```python
from build123d import *

# Parameters (mm, degrees)
F0_W          = 30.48
F0_H          = 15.24
F1_DEPTH      = 88.9
F2_W          = 30.48
F2_H          = 15.24
F3_DEPTH      = 38.1
F4_W          = 30.48
F4_H          = 15.24
F5_DEPTH      = 38.1
F6_R          = 3.81
F7_DEPTH      = 127
F7_DEPTH_BACK = 38.1
F9_DEPTH      = 88.9
F10_W         = 66.04
F10_H         = 73.66
F11_DEPTH     = 25.4
F12_W         = 63.5
F12_H         = 25.4
F13_DEPTH     = 12.7
F15_W         = 76.2
F15_H         = 25.4
F16_DEPTH     = 50.8
F18_DEPTH     = 7.62
F19_W         = 26.801726786
F19_H         = 6.35
F14_W         = 25.4
F14_H         = 6.35
F20_DEPTH     = 12.7
F21_DEPTH     = 12.7
F22_W         = 50.8
F22_H         = 25.4
F23_DEPTH     = 38.1
F24_DEPTH     = 12.7


# Not quite as in the source:
# - a feature names something its author has since deleted; it is built from what else it names


with BuildPart() as f1:
    # F0 (on Front) → F1 (new body)
    with BuildSketch(Plane.XZ):
        Polygon((0, 50.8), (0, 0), (29.5417681336, 0), (29.5417681336, 15.24), (60.0217681336, 15.24), (60.0217681336, 0), (121.1203709245, 0), (121.1203709245, 15.24), (151.6003709245, 15.24), (151.6003709245, 0), (203.2, 0), (203.2, 41.0980633142), (127, 41.0980633142), (127, 79.1980633142), (63.5, 79.1980633142), (38.1, 50.8), align=None)
        with Locations((44.7817681336, 7.62)):
            Rectangle(F0_W, F0_H)
        with Locations((136.3603709245, 7.62)):
            Rectangle(F0_W, F0_H)
    extrude(amount=F1_DEPTH)

    # F2 (on face) → F3 (cut)
    with BuildSketch(Plane.XZ.offset(88.9)):
        with Locations((45.8910012597, 7.62)):
            Rectangle(F2_W, F2_H)
        with Locations((127.1710012597, 7.62)):
            Rectangle(F2_W, F2_H)
    extrude(amount=-F3_DEPTH, mode=Mode.SUBTRACT)

    # F4 (on face) → F5 (cut)
    with BuildSketch(Plane(origin=(0, 0, 0), x_dir=(-1, 0, 0), z_dir=(0, 1, 0))):
        with Locations((-126.0602, 7.62)):
            Rectangle(F4_W, F4_H)
        with Locations((-44.7802, 7.62)):
            Rectangle(F4_W, F4_H)
    extrude(amount=-F5_DEPTH, mode=Mode.SUBTRACT)

    # F6 (on Front) → F7 (join, two sides)
    with BuildSketch(Plane.XZ) as f7_sk:
        with Locations((53.3541933731, 7.3445781872)):
            Circle(F6_R)
        with Locations((117.9336786941, 6.9635785541)):
            Circle(F6_R)
    extrude(amount=F7_DEPTH)
    extrude(f7_sk.sketch, amount=-F7_DEPTH_BACK)

    # F8 (on Front) → F9 (cut)
    with BuildSketch(Plane.XZ):
        Polygon((69.4312418273, 74.989986462), (44.0312418273, 46.5919231478), (82.1312418273, 46.5919231478), (82.1312418273, 74.989986462), align=None)
    extrude(amount=F9_DEPTH, mode=Mode.SUBTRACT)

    # F10 (on face) → F11 (cut)
    with BuildSketch(Plane.XY.offset(41.0980633142)):
        with Locations((160.02, -44.45)):
            Rectangle(F10_W, F10_H)
    extrude(amount=-F11_DEPTH, mode=Mode.SUBTRACT)

    # F12 (on face) → F13 (cut)
    with BuildSketch(Plane(origin=(-4.0760562793, 0, 3.6457355683), x_dir=(0, -1, 0), z_dir=(-0.7453559925, 0, 0.6666666667))):
        with Locations((43.8565216027, 81.8850251743)):
            Rectangle(F12_W, F12_H)
    extrude(amount=-F13_DEPTH, mode=Mode.SUBTRACT)

    # F15 (on face) → F16 (cut)
    with BuildSketch(Plane.YZ.offset(127)):
        with Locations((-44.45, 60.8695521951)):
            Rectangle(F15_W, F15_H)
    extrude(amount=-F16_DEPTH, mode=Mode.SUBTRACT)

    # F17 (on face) → F18 (join)
    with BuildSketch(Plane(origin=(0, 0, 0), x_dir=(0, -1, 0), z_dir=(-1, 0, 0))):
        Polygon((56.9462627172, 26.2763872743), (56.9462627172, 31.5944552422), (37.3661071062, 31.5944552422), (37.3661071062, 26.0346587747), (24.7961338609, 26.0346587747), (27.4551659822, 18.7827479094), (37.6078411937, 18.7827479094), (37.6078411937, 13.9481425285), (56.7045323551, 13.9481425285), (56.7045323551, 18.7827479094), (68.0658593774, 18.7827479094), (63.7147128582, 26.2763872743), align=None)
    extrude(amount=-F18_DEPTH)

    # F19 (on face) + F14 (on face) → F20 (join)
    with BuildSketch(Plane(origin=(0, 0, 0), x_dir=(0, -1, 0), z_dir=(-1, 0, 0))):
        with Locations((70.2801537674, 38.6348730328)):
            Rectangle(F19_W, F19_H)
    with BuildSketch(Plane(origin=(0, 0, 0), x_dir=(0, -1, 0), z_dir=(-1, 0, 0))):
        with Locations((18.7792903744, 38.6348730328)):
            Rectangle(F14_W, F14_H)
    extrude(amount=F20_DEPTH)

    # F21 (cut): faces of the model
    f21_faces = [f1.faces().sort_by_distance(p)[0] for p in [
        (-12.7, -18.7792903744, 38.6348730328),
        (-12.7, -70.2801537674, 38.6348730328),
    ]]
    extrude(f21_faces, amount=-F21_DEPTH, mode=Mode.SUBTRACT)

    # F22 (on face) → F23 (join)
    with BuildSketch(Plane.YZ.offset(127)):
        with Locations((-45.72, 28.3980633142)):
            Rectangle(F22_W, F22_H)
    extrude(amount=F23_DEPTH)

    # F24 (cut): a face of the model
    f24_faces = [f1.faces().sort_by_distance(p)[0] for p in [
        (165.1, -45.72, 28.3980633142),
    ]]
    extrude(f24_faces, amount=-F24_DEPTH, mode=Mode.SUBTRACT)


solid = f1.part
```
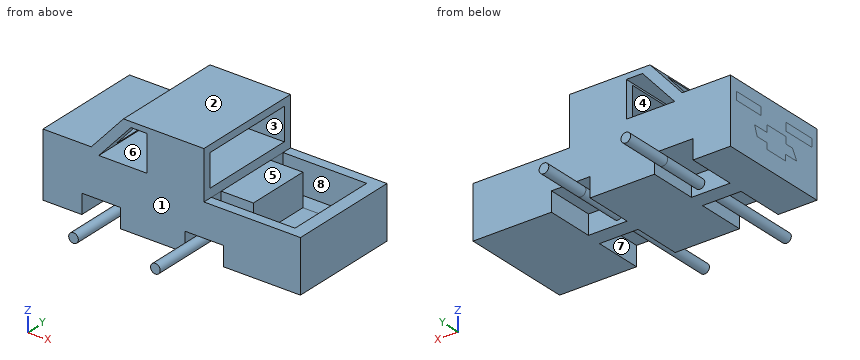
Can you work these out from the model? Positions are in its coordinate system, mm. Face numbers are marked on the shaded views. A direction names the side the tool comes from. Coordinates: 2 decimals unless noted, no trailing zeros. Order: outer loops, then holes, each group sorted by start corner. A loop starts at its lowest first (then second) coordinate and runs counter-clockwise, first axis right, second up. Notation, with made-up numbers: (48.5, 3.25) - (52.5, 3.25) arc R28 cw to (52.5, 26.25) - close; hole circle Ø2 at (37.5, 57.5). An arc over 180 degrees is marked (long way). Answer in a Markdown table with one row per item.
1. If I drill on line 1 along X through (y, z) = (-47.5, 39); line 2 along X through (y, z) = (-30, 14.5); line 3 along X through (y, z) = (-12.5, 8), over which ranges is the centre line in solid material (lowest first)?
Reply:
| item | result |
|---|---|
| line 1 | x = 0 to 152.4, 193.04 to 203.2 |
| line 2 | x = 0 to 29.54, 60.02 to 110.82, 141.3 to 203.2 |
| line 3 | x = 0 to 29.54, 49.6 to 57.11, 60.02 to 110.82, 114.27 to 121.6, 141.3 to 203.2 |
2. Suppose I cut it at D-D (y = 4). Please give me the cut outline in (x, z).
Reply:
| item | result |
|---|---|
| outline | circle Ø7.62 at (53.35, 7.34); circle Ø7.62 at (117.93, 6.96) |
3. Suppose I cut it at B-B (y = -46.5). Please give me the cut outline in (x, z), and give its area (3 significant figures).
Reply:
| item | result |
|---|---|
| outline | (0, 0) - (203.2, 0) - (203.2, 41.1) - (193.04, 41.1) - (193.04, 15.7) - (152.4, 15.7) - (152.4, 41.1) - (127, 41.1) - (127, 48.17) - (82.13, 48.17) - (82.13, 46.59) - (44.03, 46.59) - (47.43, 50.4) - (42.05, 55.21) - (38.1, 50.8) - (0, 50.8) - close; (58.98, 74.15) - (64.37, 69.33) - (69.43, 74.99) - (82.13, 74.99) - (82.13, 73.57) - (127, 73.57) - (127, 79.2) - (63.5, 79.2) - close |
| area | 8,670 mm^2 |
4. Suppose I cut it at C-C (x = 26). Please give me the cut outline in (y, z).
Reply:
| item | result |
|---|---|
| outline | (-88.9, 0) - (0, 0) - (0, 50.8) - (-88.9, 50.8) - close |
5. For pin 1 (24.5 mm diameter, centred on x = 43.5, y = -12, fed in from -Z); pin 2 (24.5 mm diameter, centred on x = 54, z = 58, fed in from -Y); pin 3 (8 mm diameter, centred on x = 132, y = -8.5, fed in from -Z), each with a flat end and sliding along its axis, tell me the tip position at first contact or that it passes through.
Reply:
| item | result |
|---|---|
| pin 1 | stops at z = 3.53 |
| pin 2 | stops at y = -88.9 |
| pin 3 | stops at z = 15.24 |
6. Suppose I cut it at A-A (x = 95.5). Please give me the cut outline in (y, z), and give its area (3 significant figures).
Reply:
| item | result |
|---|---|
| outline | (-88.9, 0) - (0, 0) - (0, 79.2) - (-88.9, 79.2) - close; hole (-82.55, 48.17) - (-6.35, 48.17) - (-6.35, 73.57) - (-82.55, 73.57) - close |
| area | 5,110 mm^2 |
7. For the marked faces 5, 6, 7 and 8, which set-ups out of +Z, -Z, +X, -X, +Y, -Y let a thin tool reach every point of the face, with its end or its side?
Reply:
| item | result |
|---|---|
| face 5 | +Z, +X, +Y, -Y |
| face 6 | +Y, -Y |
| face 7 | -Z, -Y |
| face 8 | +Z |
8. If we mould it in two halves opening along Z, with no side actions, what happens to the marked faces 1, 2, 3 and 4? For each: pulls with the +Z half, pulls with the -Z half, needs draft (parallel to the pull), parting line crosses it, or undercut.
Reply:
| item | result |
|---|---|
| face 1 | needs draft |
| face 2 | pulls with the +Z half |
| face 3 | undercut |
| face 4 | undercut |
